Job drawing, mm, ordinate dimensions from the low corner. One solid piece. A direction names the side the tool comes from. Give positions to 0.01 mm unless a question says otherwise; leave off trailing zeros. Loops run counter-clockwise (first coordinate to the right, second up) from the corner with the lowest first, then second, coordinate; pieces in that order, holes last. Notation, with made-up numbers: (-22.75, 67.25) -> (-13.75, 67.25) arc R21 cw to (-13.75, 77.25) -> close; hole circle Ø10 at (52, 5). An arc over 180 degrees is marked (long way). Answer as a JSON object with one key per item and string values. Group by question number.
Q1. Band-saw the part on C-C, the plane y = 7.5. Write the cut outline in (x, z), plus the area to 3 significant figures.
Q2. Band-saw the part on B-B, the plane x = 34. Write the cut outline in (y, z), plus the area to 3 significant figures.
Q3. Band-saw the part on A-A, the plane z = 34. Write the cut outline in (x, y), plus the area to 3 significant figures.
Q4. Wall check: probe 1 along Z at (x, y) = (34, 3.75); probe 2 along Z at (x, y) = (59, 7.5); probe 3 along X at (y, z) = (12.25, 35). Give the ranges that are in metal, low to high. Write a range as from..to.
Q5. Tool access for the marked faces 4 and 5: list every direction of +Z, -Z, +X, -X, +Y, -Y with a clear straight run to the whole face (end or side of a thin tool).
Q6. Drop flat-ended pins along their axis: pin 1 (3 mm diameter, centred on x = 28.5, y = 7, fed in from +Z); pin 2 (8 mm diameter, centred on y = 7, z = 58.5, fed in from -X); pin 3 (4 mm diameter, centred on x = 19.5, y = 7.5, fed in from -Z). Give the stop position or say it passes through.
Q7. Two-plate mould, pull along X, no slides. Class the marked faces 1, 2 and 3: pulls with the +X half, pulls with the -X half, needs draft (parallel to the pull), parting line crosses it, or undercut.
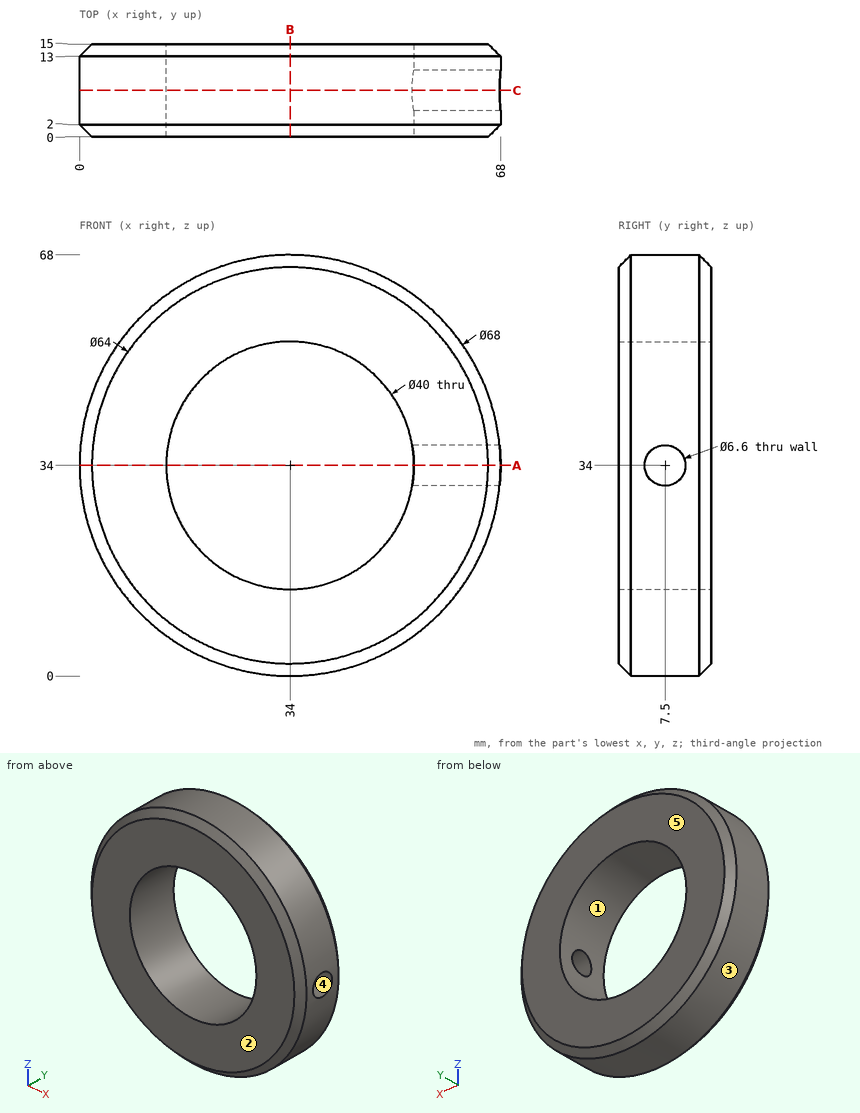
Worked answers:
{
 "1": {"outline": "(53.73, 30.7) arc R20 cw (long way) to (53.73, 37.3) -> (67.84, 37.3) arc R34 ccw (long way) to (67.84, 30.7) -> close", "area": "2,280 mm2"},
 "2": {"outline": "(0, 2) -> (2, 0) -> (13, 0) -> (15, 2) -> (15, 14) -> (0, 14) -> close; (0, 54) -> (15, 54) -> (15, 66) -> (13, 68) -> (2, 68) -> (0, 66) -> close", "area": "412 mm2"},
 "3": {"outline": "(0, 2) -> (2, 0) -> (14, 0) -> (14, 15) -> (2, 15) -> (0, 13) -> close; (54, 0) -> (66, 0) -> (68, 2) -> (68, 4.2) -> (54, 4.2) -> close; (54, 10.8) -> (68, 10.8) -> (68, 13) -> (66, 15) -> (54, 15) -> close", "area": "320 mm2"},
 "4": {"probe 1": "0..14, 54..68", "probe 2": "10.96..30.7, 37.3..57.04", "probe 3": "0.01..14.03, 53.97..67.99"},
 "5": {"face 4": "+X", "face 5": "+Z, -Z, +X, -X, +Y"},
 "6": {"pin 1": "z = 67.76", "pin 2": "x = 6.88", "pin 3": "z = 2.38"},
 "7": {"face 1": "undercut", "face 2": "needs draft", "face 3": "parting line crosses it"}
}
